Verification items for this drawing (mm, ordinates from the low corner). Round coordinates to 2 decimals unless told otherwise and drop trailing zeros. Write each loop counter-clockwise with the first axis right and the second up, starting at its lowest first coordinate (ties: lowest second). Pieces come first, ordered by that corner, then holes. Notation, with made-up numbers: (-39.75, -9.5) - (-26.75, -9.5) arc R16 cw to (-26.75, 1.5) - close; hole circle Ø4 at (-19.5, 60). An arc over 180 degrees is marked (long way). One line per question, with ' | ' between items. Start each with the question number.
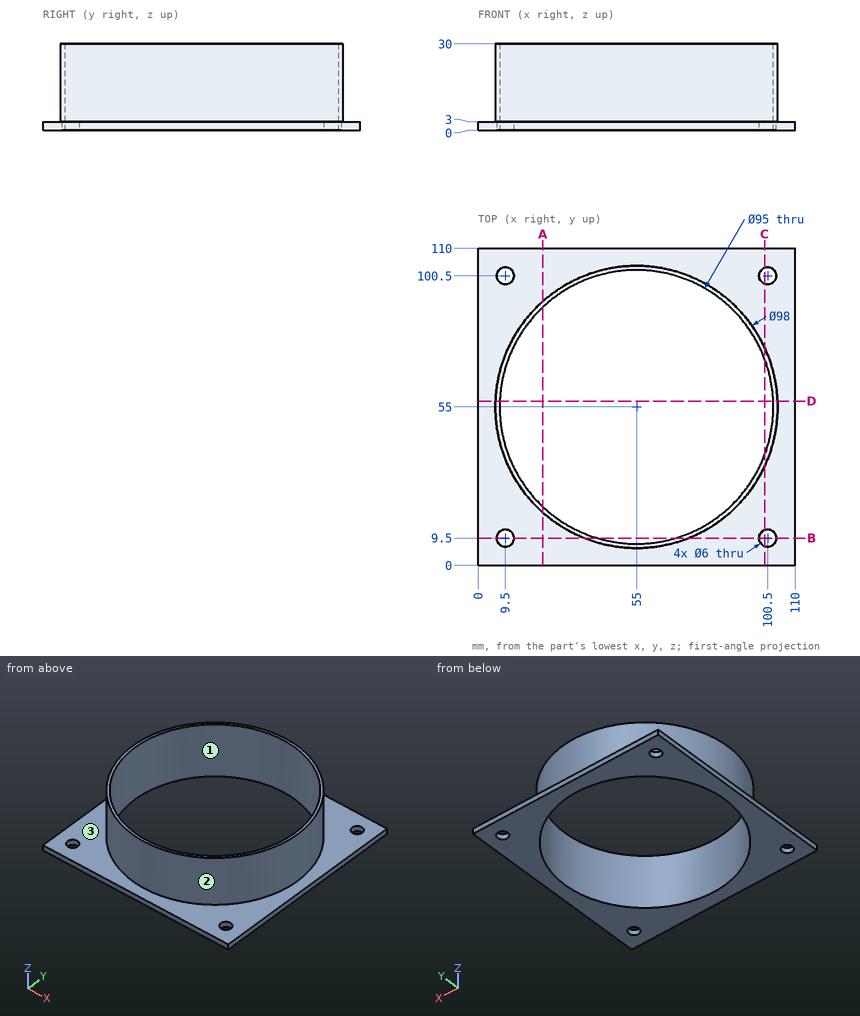
Q1. Thickness scan on line 1 (Y direction, x = 55, z = 13.5); line 2 (X direction, y = 54, z = 4.5); line 3 (Y direction, x = 48, z = 11.25). Record the ranges inside material, lowest first.
Q2. Section check D-D, the plane y = 57. Record the cut outline in (x, z), then the cut area to 3 significant figures.
Q3. Section check A-A, the plane x = 22.5. Record the cut outline in (y, z).
Q4. Section check C-C, the plane x = 99.5. Record the cut outline in (y, z).
Q5. Section check B-B, the plane y = 9.5. Record the cut outline in (x, z).
Q6. Draft check along Y on the marked faces 1, 2 and 3. Enter one of: pulls with the +Y half, pulls with the -Y half, needs draft (parallel to the pull), parting line crosses it, or undercut.
Q7. Go/stop test with flat-tipped pins: P1, Ø1.5, axis at x = 37.5, z = 6, coming from the -Y side; P2, Ø6, axis at y = 51.5, z = 24.5, coming from the +X side; P3, Ø3, axis at y = 29.5, z = 25, coming from the +X side; P4, Ø5.5, axis at x = 100.5, y = 9.5, coming from the -Z side. Record where each tip stops, or that it passes through.
Result sheet:
1) line 1: 6 to 7.5, 102.5 to 104 | line 2: 6.01 to 7.51, 102.49 to 103.99 | line 3: 6.5 to 8.02, 101.98 to 103.5
2) outline: (0, 0) - (7.54, 0) - (7.54, 30) - (6.04, 30) - (6.04, 3) - (0, 3) - close; (102.46, 0) - (110, 0) - (110, 3) - (103.96, 3) - (103.96, 30) - (102.46, 30) - close | area: 126 mm²
3) outline: (0, 0) - (20.36, 0) - (20.36, 30) - (18.33, 30) - (18.33, 3) - (0, 3) - close; (89.64, 0) - (110, 0) - (110, 3) - (91.67, 3) - (91.67, 30) - (89.64, 30) - close
4) outline: (0, 0) - (6.67, 0) - (6.67, 3) - (0, 3) - close; (12.33, 0) - (38.39, 0) - (38.39, 30) - (34.49, 30) - (34.49, 3) - (12.33, 3) - close; (71.61, 0) - (97.67, 0) - (97.67, 3) - (75.51, 3) - (75.51, 30) - (71.61, 30) - close; (103.33, 0) - (110, 0) - (110, 3) - (103.33, 3) - close
5) outline: (0, 0) - (6.5, 0) - (6.5, 3) - (0, 3) - close; (12.5, 0) - (41.36, 0) - (41.36, 30) - (36.81, 30) - (36.81, 3) - (12.5, 3) - close; (68.64, 0) - (97.5, 0) - (97.5, 3) - (73.19, 3) - (73.19, 30) - (68.64, 30) - close; (103.5, 0) - (110, 0) - (110, 3) - (103.5, 3) - close
6) face 1: undercut | face 2: parting line crosses it | face 3: needs draft
7) P1: y = 8.95 | P2: x = 104 | P3: x = 97.72 | P4: through
